Geometry check sheet. Reference: the model listing, model coordinates, mm. A direction names the side the tool comes from. Round coordinates to 2 decimals unless told otherwise and drop trailing zeros. Loops run counter-clockwise (first coordinate to the right, second up) from the corner with the lowest first, then second, coordinate; pieces in that order, holes last. Notation, with made-up numbers: M 48.5,-1 L 99.5,-1 A28 ccw 99.5,27 Z; hole C 67,-29.75 d4. An arc over 180 degrees is marked long. Write item = value, one per line.
Autodesk Inventor part; units mm, degrees
ref_plane "Płaszczyzna konstrukcyjna1" through (0, 0, 0) normal (0, 0, 1) x (1, 0, 0)
ref_plane "YZ Plane" through (0, 0, 0) normal (1, 0, 0) x (0, 1, 0)
ref_plane "XZ Plane" through (0, 0, 0) normal (0, 1, 0) x (-1, 0, 0)
ref_plane "Płaszczyzna konstrukcyjna1" through (0, 0, 0) normal (0, 0, 1) x (1, 0, 0)
sketch "Szkic1" plane through (0, 0, 0) normal (0, 0, 1) x (1, 0, 0)
  circle A0 centre (-0.75, -19.05) radius 2
  circle A1 centre (-0.75, 1.9) radius 2
  circle A2 centre (-53.2, 1.9) radius 2
  circle A3 centre (-53.2, -19.05) radius 2
  arc A4 (-7.07, 6.8616) -> (-7.3, 7.3) centre (-6.1, 7.65) ccw
  line L0 (-7.07, 6.8616) -> (-7.07, -24.52)
  line L1 (-7.07, -24.52) -> (-47.8, -24.52)
  line L2 (-47.8, -24.52) -> (-47.8, 7.3)
  line L3 (-47.8, 7.3) -> (-7.3, 7.3)
  arc A5 (-49.8576, -25.4424) -> (-50.3424, -24.9576) centre (-49.25, -24.35) ccw
  line L4 (-49.8576, -25.4424) -> (-47.9, -27.4)
  line L5 (-47.9, -27.4) -> (-33.9, -27.4)
  line L6 (-33.9, -27.4) -> (-30.0895, -29.6)
  line L7 (-30.0895, -29.6) -> (-13.35, -29.6)
  line L8 (-13.35, -29.6) -> (-11.15, -27.4)
  line L9 (-11.15, -27.4) -> (-7.15, -27.4)
  line L10 (-7.15, -27.4) -> (-2.65, -22.9)
  line L11 (-2.65, -22.9) -> (-2.65, 6.4)
  line L12 (-2.65, 6.4) -> (-6.65, 10.4)
  line L13 (-6.65, 10.4) -> (-47.9, 10.4)
  arc A6 (-47.9, 10.4) -> (-50.9, 7.4) centre (-47.9, 7.4) ccw
  line L14 (-50.9, 7.4) -> (-50.9, -24.4)
  line L15 (-50.9, -24.4) -> (-50.3424, -24.9576)
  line L16 (-50.3424, -24.9576) -> (-49.8576, -25.4424)
  arc A7 (-49.8576, -25.4424) -> (-50.3424, -24.9576) centre (-49.25, -24.35) ccw
  line L17 (-42.875, -20.03) -> (-42.875, 2.83)
  line L18 (-42.875, 2.83) -> (-12.075, 2.83)
  line L19 (-12.075, 2.83) -> (-12.075, -20.03)
  line L20 (-12.075, -20.03) -> (-42.875, -20.03)
  line L21 (-45.382, -22.57) -> (-9.568, -22.57)
  line L22 (-9.568, -22.57) -> (-9.568, 5.37)
  line L23 (-9.568, 5.37) -> (-45.382, 5.37)
  line L24 (-45.382, 5.37) -> (-45.382, -22.57)
  arc A8 (-18.975, -17.3) -> (-14.775, -13.1) centre (-18.975, -13.1) ccw
  line L25 (-18.975, -17.3) -> (-35.975, -17.3)
  arc A9 (-40.175, -13.1) -> (-35.975, -17.3) centre (-35.975, -13.1) ccw
  line L26 (-40.175, -13.1) -> (-40.175, -4.1)
  arc A10 (-35.975, 0.1) -> (-40.175, -4.1) centre (-35.975, -4.1) ccw
  line L27 (-35.975, 0.1) -> (-18.975, 0.1)
  arc A11 (-14.775, -4.1) -> (-18.975, 0.1) centre (-18.975, -4.1) ccw
  line L28 (-14.775, -4.1) -> (-14.775, -13.1)
  line L29 (-42.875, -20.03) -> (-12.075, -20.03)
  line L30 (-12.075, -20.03) -> (-12.075, 2.83)
  line L31 (-12.075, 2.83) -> (-42.875, 2.83)
  line L32 (-42.875, 2.83) -> (-42.875, -20.03)
  line L33 (-62.5, -30.65) -> (-6.9, -30.65) construction
  line L34 (-62.5, 29.05) -> (-62.5, -29.05)
  line L35 (-62.5, -29.05) -> (8.2, -29.05)
  circle A12 centre (-0.75, -19.05) radius 1.25
  circle A13 centre (-0.75, 1.9) radius 1.25
  circle A14 centre (-53.2, 1.9) radius 1.25
  circle A15 centre (-53.2, -19.05) radius 1.25
  circle A16 centre (-49.25, -24.35) radius 1.3
  circle A17 centre (-6.1, 7.65) radius 1.3
  line L36 (-11.575, -20.53) -> (-43.375, -20.53)
  line L37 (-43.375, -20.53) -> (-43.375, 3.33)
  line L38 (-43.375, 3.33) -> (-11.575, 3.33)
  line L39 (-11.575, 3.33) -> (-11.575, -20.53)
  line L40 (-27.475, -20.03) -> (-27.475, 2.83) construction
  line L41 (-11.575, -8.6) -> (-43.375, -8.6) construction
  line L42 (2.525, -38.6) -> (-57.475, -38.6) construction
  line L43 (-57.475, -38.6) -> (-57.475, 21.4) construction
  line L44 (-57.475, 21.4) -> (2.525, 21.4) construction
  line L45 (2.525, 21.4) -> (2.525, -38.6) construction
  line L46 (2.525, -38.6) -> (-57.475, 21.4) construction
  line L47 (-57.475, -38.6) -> (2.525, 21.4) construction
  line L48 (10.025, -46.1) -> (-64.975, -46.1)
  line L49 (-64.975, -46.1) -> (-64.975, 28.9)
  line L50 (-64.975, 28.9) -> (10.025, 28.9)
  line L51 (10.025, 28.9) -> (10.025, -46.1)
  line L52 (10.025, -46.1) -> (-64.975, 28.9) construction
  line L53 (-64.975, -46.1) -> (10.025, 28.9) construction
  circle A18 centre (-57.475, 21.4) radius 3
  circle A19 centre (2.525, 21.4) radius 3
  circle A20 centre (2.525, -38.6) radius 3
  circle A21 centre (-57.475, -38.6) radius 3
  line L54 (-2.35, -32.15) -> (-51.2, -32.15)
  line L55 (-51.2, -32.15) -> (-51.2, 10.7)
  line L56 (-51.2, 10.7) -> (-2.35, 10.7)
  line L57 (-62.5, -32.15) -> (147.5, -32.15)
  circle A22 centre (-0.75, 1.9) radius 1.5 construction
  line L58 (-2.35, 3.1) -> (-2.65, 2.5245)
  line L59 (-2.65, 2.5245) -> (-2.65, 1.2755)
  line L60 (-2.65, 1.2755) -> (-2.35, 0.7)
  line L61 (-2.35, -17.85) -> (-2.65, -18.4255)
  line L62 (-2.65, -18.4255) -> (-2.65, -19.6745)
  line L63 (-2.65, -19.6745) -> (-2.35, -20.25)
  line L64 (-2.35, -20.25) -> (-2.35, -32.15)
  line L65 (-2.35, 10.7) -> (-2.35, 3.1)
  line L66 (-2.35, 0.7) -> (-2.35, -17.85)
  point P0 (0, 0)
  point P1 (-27.475, -8.6)
  dimension "d0" = 2.5
  dimension "d1" = 2.6
  dimension "d2" = 2.6
  dimension "d3" = 0.5
  dimension "d4" = 0.5
  dimension "d5" = 0.5
  dimension "d6" = 0.5
  dimension "d7" = 60
  dimension "d8" = 75
  dimension "d9" = 6
  dimension "d10" = 0.3
  dimension "d12" = 0.3
  dimension "d36" = 3
  dimension "d37" = 0.3
extrude "Wyciągnięcie proste1" add sketch "Szkic1" along normal blind 15 contours A0 L63 L11 L61 | A3 | A2 | A0 L66 A1 L65 L56 L55 L35 L34 L50 L51 L57 L64 | L61 A0 | A0 L11 A1 L66 | L64 L35 L8 L9 L10 L11 A0 | A0 L63 | L11 A0 | A0 L11 L10 L9 L8 L35 L6 L5 L4 A16 L15 L14 A6 L13 L12 A1 | L60 L11 L58 A1 | A1 L60 | L64 L54 L55 L35 L6 L7 L8 | A1 L11 | L8 L7 L6 L35 | L57 L51 L48 L49 L50 L34 L35 L55 L54 | L11 L12 L13 A6 L14 L15 A16 L4 L5 L6 L35 L55 L56 L65 A1 | A1 L58 | L0 L1 L2 L3 A17 | L24 L23 L22 L21
sketch "Szkic2" plane through (0, 0, 0) normal (0, 0, -1) x (-1, 0, 0)
  line L0 (64.975, 28.9) -> (64.975, -46.1)
  line L1 (-10.025, 28.9) -> (64.975, 28.9)
  line L2 (-10.025, -46.1) -> (-10.025, 28.9)
  line L3 (64.975, -46.1) -> (-10.025, -46.1)
  line L4 (11.575, -20.53) -> (43.375, -20.53)
  line L5 (11.575, 3.33) -> (11.575, -20.53)
  line L6 (43.375, 3.33) -> (11.575, 3.33)
  line L7 (43.375, -20.53) -> (43.375, 3.33)
  circle A0 centre (49.25, -24.35) radius 1.3
  circle A1 centre (57.475, -38.6) radius 3
  circle A2 centre (-2.525, -38.6) radius 3
  circle A3 centre (-2.525, 21.4) radius 3
  circle A4 centre (57.475, 21.4) radius 3
  circle A5 centre (0.75, 1.9) radius 1.25
  circle A6 centre (0.75, -19.05) radius 1.25
  circle A7 centre (53.2, -19.05) radius 1.25
  circle A8 centre (53.2, 1.9) radius 1.25
  circle A9 centre (6.1, 7.65) radius 1.3
  line L8 (6.65, 10.4) -> (47.9, 10.4)
  arc A10 (50.9, 7.4) -> (47.9, 10.4) centre (47.9, 7.4) ccw
  line L9 (50.9, 7.4) -> (50.9, -24.4)
  line L10 (2.65, 6.4) -> (6.65, 10.4)
  line L11 (2.65, -22.9) -> (2.65, 6.4)
  line L12 (7.15, -27.4) -> (2.65, -22.9)
  line L13 (11.15, -27.4) -> (7.15, -27.4)
  line L14 (13.35, -29.6) -> (11.15, -27.4)
  line L15 (50.9, -24.4) -> (47.9, -27.4)
  line L16 (47.9, -27.4) -> (33.9, -27.4)
  line L17 (33.9, -27.4) -> (30.0895, -29.6)
  line L18 (30.0895, -29.6) -> (13.35, -29.6)
  line L19 (2.25, 10.7) -> (51.1, 10.7)
  line L20 (51.1, 10.7) -> (51.1, -34.4144)
  line L21 (51.1, -34.4144) -> (2.25, -34.4144)
  line L22 (62.5, -30.65) -> (6.9, -30.65) construction
  line L23 (62.5, -32.15) -> (-147.5, -32.15) construction
  circle A11 centre (0.75, 1.9) radius 1.5 construction
  circle A12 centre (0.75, -19.05) radius 1.5 construction
  line L24 (2.6, 3.4) -> (2.6, 0.4)
  line L25 (2.6, 0.4) -> (2.25, 0.05)
  line L26 (2.6, 3.4) -> (2.25, 3.75)
  line L27 (2.25, -17.2) -> (2.6, -17.55)
  line L28 (2.6, -17.55) -> (2.6, -20.55)
  line L29 (2.6, -20.55) -> (2.25, -20.9)
  line L30 (2.25, 3.75) -> (2.25, 10.7)
  line L31 (2.25, -34.4144) -> (2.25, -20.9)
  line L32 (2.25, -17.2) -> (2.25, 0.05)
  point P0 (0, 0)
  point P1 (2.6, 1.9)
  point P2 (2.6, -19.05)
  dimension "d15" = 0.2
  dimension "d16" = 0.3
  dimension "d38" = 3
  dimension "d39" = 3
  dimension "d40" = 3
  dimension "d41" = 3
  dimension "d43" = 0.05
  dimension "d44" = 48.85
  dimension "d45" = 45
  dimension "d46" = 45
extrude "Wyciągnięcie proste2" cut sketch "Szkic2" against normal blind 4.33 contours A0 L15 L16 L17 L18 L14 L13 L12 L11 L10 L8 A10 L9 | L19 L20 L21 L31 L29 L28 L27 L32 L25 L24 L26 L30
sketch "Szkic3" plane through (-64.975, -46.1, 0) normal (-1, 0, 0) x (0, 0, 1)
  line L0 (0, 75) -> (0, 0)
  line L1 (0, 0) -> (15, 0)
  line L2 (0, 15.45) -> (7.3, 15.45)
  line L3 (7.3, 15.45) -> (7.3, 0)
  line L4 (7.3, 0) -> (0, 0)
  line L5 (0, 0) -> (0, 15.45)
  line L6 (-98.1, 15.45) -> (7, 15.45)
  line L7 (7, 15.45) -> (7, 13.95)
  line L8 (-98.1, 13.95) -> (7, 13.95)
  line L9 (-98.1, 15.45) -> (-98.1, 13.95)
  point P0 (0, 46.1)
  dimension "d22" = 0.3
extrude "Wyciągnięcie proste3" cut sketch "Szkic3" against normal up to next contours L2 L7 L8 L0 | L8 L7 L2 L3 L1 L0
chamfer "Faza1" distance 2.5 angle 45 4 edges at (-64.975, 28.9, 7.5) (-64.975, -46.1, 11.15) (10.025, -46.1, 11.15) (10.025, 28.9, 7.5)
sketch "Szkic4" plane through (0, 0, 0) normal (0, 0, -1) x (-1, 0, 0)
  line L0 (-8.5, -30.65) -> (-64.1, -30.65) construction
  line L1 (-8.5, -30.65) -> (-8.5, -22.05) construction
  line L2 (-64.1, -22.05) -> (-8.5, -22.05) construction
  line L3 (-64.1, -30.65) -> (-64.1, -22.05) construction
  line L4 (-10.025, -30.65) -> (-10.025, 26.4)
  line L5 (-10.025, -30.65) -> (-6.5, -30.65)
  line L6 (-6.5, -30.65) -> (-6.5, -21.05)
  line L7 (-6.5, -21.05) -> (-10.025, -21.05)
  line L8 (-10.025, -21.05) -> (-10.025, -30.65)
  point P0 (0, 0)
  point P1 (-8.2625, -21.05)
  dimension "d26" = 1
  dimension "d27" = 2
extrude "Wyciągnięcie proste4" cut sketch "Szkic4" against normal up to surface (7.3 mm away)
sketch "Szkic6" plane through (0, 0, 15) normal (0, 0, 1) x (1, 0, 0)
  circle A0 centre (-57.475, -38.6) radius 3 construction
  circle A1 centre (2.525, -38.6) radius 3 construction
  line L0 (-57.475, -38.6) -> (2.525, -38.6) construction
  circle A2 centre (-42.475, -38.6) radius 1.25
  circle A3 centre (-12.475, -38.6) radius 1.25
  point P0 (0, 0)
  dimension "d30" = 2.5
  dimension "d31" = 15
  dimension "d32" = 2.5
  dimension "d33" = 15
extrude "Wyciągnięcie proste5" cut sketch "Szkic6" against normal up to next
properties part number "mocowanie_2000"
(1) Sectioned sample at A-A on x = -49.25. Record the cut outline in (y, z).
Result set:
outline = M -46.1,7.3 L -30.65,7.3 L -30.65,4.33 L -25.65,4.33 L -25.65,15 L -46.1,15 Z; M -23.05,4.33 L 10.7,4.33 L 10.7,0 L 28.9,0 L 28.9,15 L -23.05,15 Z
(2) Sectioned sample at C-C on z = 1.5. Record the cut outline in (x, y) (3 decimals).
Result set:
outline = M -64.975,-30.65 L -51.1,-30.65 L -51.1,10.7 L -2.25,10.7 L -2.25,3.75 L -2.6,3.4 L -2.6,0.4 L -2.25,0.05 L -2.25,-17.2 L -2.6,-17.55 L -2.6,-20.55 L -2.25,-20.9 L -2.25,-30.65 L 6.5,-30.65 L 6.5,-21.05 L 10.025,-21.05 L 10.025,26.4 L 7.525,28.9 L -62.475,28.9 L -64.975,26.4 Z; hole C -57.475,21.4 d6; hole C -53.2,-19.05 d2.5; hole C -53.2,1.9 d2.5; hole C -0.75,-19.05 d2.5; hole C -0.75,1.9 d2.5; hole C 2.525,21.4 d6
(3) Release check for a two-part mould opening along Y. For faces 1 (the flat face through (8, -21.05, 4)), 2 (the flat face through (-2.25, 7, 2)), 3 (the flat face through (10.025, 0, 7)) record: released by +Y, released by -Y, zero draft, split by the parting line, or undercut.
Result set:
face_1 = released by -Y
face_2 = undercut
face_3 = zero draft
(4) Tool access check on faces 4 (the flat face through (-51.1, -10, 2)), 5 (the flat face through (-28, 13, 0)), 6 (the flat face through (-11.575, -8, 10)). Record the directions out of +Z, -Z, +X, -X, +Y, -Y that give a thin tool (end or side, any length) a straight path to the whole face; none if there is none.
Result set:
face_4 = -Z, -Y
face_5 = -Z, +X, -X, +Y, -Y
face_6 = +Z, -Z
(5) Material ranges on line 1 along X through (y, z) = (-12.5, 6.5) (3 decimals); line 2 along X through (y, z) = (-5.5, 1) (3 decimals); line 3 along Y through (x, z) = (-53.2, 3.25), recorded low to high. Write a range as from..to.
Result set:
line_1 = -64.975..-43.375, -11.575..10.025
line_2 = -64.975..-51.1, -2.25..10.025
line_3 = -30.65..-20.3, -17.8..0.65, 3.15..28.9
(6) Depth check by flat-ended pin: pin 1 Ø4 at (x, y) = (-43.5, -32) entering from -Z; pin 2 Ø1.3 at (x, z) = (-37, 2) entering from -Y; pin 3 Ø3.5 at (y, z) = (-25.5, 5) entering from +X. Enter the tip coordinate at first touch or a pass-through.
Result set:
pin_1 = 4.33
pin_2 = 10.7
pin_3 = 6.5
(7) Sectioned sample at B-B on y = 1.9. Record the cut outline in (x, z) (3 decimals).
Result set:
outline = M -64.975,0 L -54.45,0 L -54.45,15 L -64.975,15 Z; M -51.95,0 L -51.1,0 L -51.1,4.33 L -43.375,4.33 L -43.375,15 L -51.95,15 Z; M -11.575,4.33 L -2.6,4.33 L -2.6,0 L -2,0 L -2,15 L -11.575,15 Z; M 0.5,0 L 10.025,0 L 10.025,15 L 0.5,15 Z
(8) Sectioned sample at D-D on y = -38.6. Record the cut outline in (x, z) (3 decimals), then the cut area to 3 significant figures.
Result set:
outline = M -64.975,7.3 L -60.475,7.3 L -60.475,15 L -64.975,15 Z; M -54.475,7.3 L -43.725,7.3 L -43.725,15 L -54.475,15 Z; M -41.225,7.3 L -13.725,7.3 L -13.725,15 L -41.225,15 Z; M -11.225,7.3 L -0.475,7.3 L -0.475,15 L -11.225,15 Z; M 5.525,7.3 L 10.025,7.3 L 10.025,15 L 5.525,15 Z
area = 447 mm2
